Model file for the job. Use its own axes, mm. A direction names the side the tool comes from. Coordinates: 2 decimals unless noted, no trailing zeros. Loops run counter-clockwise (first coordinate to the right, second up) from the corner with the lowest first, then second, coordinate; pieces in that order, holes last. Notation, with made-up numbers: (-39.75, -15) -> (-34.75, -15) arc R14 cw to (-34.75, 12) -> close; hole circle Ø1 at (7.25, 77.5). An arc over 180 degrees is marked (long way). Use one line per item in the form item = value.
```python
from build123d import *

# Parameters (mm, degrees)
BOSS_EXTRUDE1_DEPTH             = 15.875
SKETCH2_R                       = 4.7625
CUT_EXTRUDE1_DEPTH              = 8
SKETCH3_R                       = 4.7625
CUT_EXTRUDE2_DEPTH              = 8
CUT_EXTRUDE3_DEPTH              = 60.905780189
BOSS_EXTRUDE2_REACH             = 62.821
BOSS_EXTRUDE2_DIRECTION_2_DEPTH = 31.75
SKETCH6_R                       = 4.7625
CUT_EXTRUDE4_DEPTH              = 83.269033521
CUT_EXTRUDE5_DEPTH              = 31.75
BOSS_EXTRUDE4_DEPTH             = 31.75
CUT_EXTRUDE6_DEPTH              = 93.319424063
BOSS_EXTRUDE5_DEPTH             = 12.7
BOSS_EXTRUDE6_DEPTH             = 6.35
CUT_EXTRUDE7_DEPTH              = 71.05833388
CUT_EXTRUDE8_REACH              = 78.805
SKETCH15_R                      = 2.25
CUT_EXTRUDE9_DEPTH              = 44.45
CUT_EXTRUDE10_DEPTH             = 12.7
SKETCH21_W                      = 12.513073453
SKETCH21_H                      = 19.05
CUT_EXTRUDE11_DEPTH             = 69.753972493


with BuildPart() as part:
    # Sketch1 → Boss-Extrude1 (new, symmetric)
    with BuildSketch(Plane(origin=(0, 0, 0), x_dir=(1, 0, 0), z_dir=(0, 1, 0))):
        Polygon((-35.921024484, 0), (0, 35.921024484), (35.921024484, 0), (0, -35.921024484), align=None)
    extrude(amount=BOSS_EXTRUDE1_DEPTH, both=True)

    # Sketch2 → Cut-Extrude1 (cut)
    with BuildSketch(Plane(origin=(17.960512242, 0, 17.960512242), x_dir=(0.7071067811865476, 0, -0.7071067811865476), z_dir=(0.7071067811865476, 0, 0.7071067811865476))):
        Circle(SKETCH2_R)
    extrude(amount=-CUT_EXTRUDE1_DEPTH, mode=Mode.SUBTRACT)

    # Sketch3 → Cut-Extrude2 (cut)
    with BuildSketch(Plane(origin=(-17.960512242, 0, 17.960512242), x_dir=(0.7071067811865472, 0, 0.7071067811865478), z_dir=(-0.7071067811865478, 0, 0.7071067811865472))):
        Circle(SKETCH3_R)
    extrude(amount=-CUT_EXTRUDE2_DEPTH, mode=Mode.SUBTRACT)

    # Sketch4 → Cut-Extrude3 (cut, through all)
    with BuildSketch(Plane(origin=(0, 15.875, 0), x_dir=(1, 0, 0), z_dir=(0, 1, 0))):
        Polygon((25.4, 10.521024484), (-25.4, 10.521024484), (0, 35.921024484), align=None)
    extrude(amount=-CUT_EXTRUDE3_DEPTH, mode=Mode.SUBTRACT)

    # Boss-Extrude2: up to this face of the body (flat: up to its plane)
    boss_extrude2_end = Plane(part.part.faces().sort_by_distance((30.660512242, 0, -5.260512242))[0])
    # Sketch5 → Boss-Extrude2 (add, up to the picked face)
    with BuildSketch(Plane(origin=(0, 0, -10.521024484), x_dir=(-1, 0, 0), z_dir=(0, 0, -1)), mode=Mode.PRIVATE) as boss_extrude2_sk1:
        Polygon((-35.921024484, 15.875), (-35.921024484, -15.875), (39.135030454, -15.875), (27.578975516, 15.875), align=None)
    boss_extrude2_tool1 = split(extrude(boss_extrude2_sk1.sketch, amount=-BOSS_EXTRUDE2_REACH, mode=Mode.PRIVATE), bisect_by=boss_extrude2_end, keep=Keep.BOTH, mode=Mode.PRIVATE)
    add(boss_extrude2_tool1.solids().sort_by(Axis((1.201693, -0.441343, -10.521024), (0, 0, 1)))[0])

    # Sketch5 → Boss-Extrude2 direction 2 (add)
    with BuildSketch(Plane(origin=(0, 0, -10.521024484), x_dir=(-1, 0, 0), z_dir=(0, 0, -1))):
        Polygon((-35.921024484, 15.875), (-35.921024484, -15.875), (39.135030454, -15.875), (27.578975516, 15.875), align=None)
    extrude(amount=BOSS_EXTRUDE2_DIRECTION_2_DEPTH)

    # Sketch6 → Cut-Extrude4 (cut, through all)
    with BuildSketch(Plane(origin=(-29.45497488, 10.720734107, 0), x_dir=(0, 0, 1), z_dir=(-0.9396926207859072, 0.3420201433256724, 0))):
        with Locations(Location((-26.396024484, -11.408766942, 0), (0, 0, 270))):
            Circle(SKETCH6_R)
    extrude(amount=-CUT_EXTRUDE4_DEPTH, mode=Mode.SUBTRACT)

    # Sketch7 → Cut-Extrude5 (cut)
    with BuildSketch(Plane(origin=(0, 0, -42.271024484), x_dir=(-1, 0, 0), z_dir=(0, 0, -1))):
        Polygon((20.821446661, 15.875), (32.377501598, -15.875), (-35.921024484, -15.875), (-35.921024484, 15.875), align=None)
    extrude(amount=-CUT_EXTRUDE5_DEPTH, mode=Mode.SUBTRACT)

    # Sketch9 → Boss-Extrude4 (add)
    with BuildSketch(Plane.XZ.offset(15.875)):
        Polygon((-25.4, -10.521024484), (-35.921024484, 0), (-46.442048969, -10.521024484), align=None)
    extrude(amount=-BOSS_EXTRUDE4_DEPTH)

    # Sketch10 → Cut-Extrude6 (cut, through all)
    with BuildSketch(Plane(origin=(0, 0, -42.271024484), x_dir=(-1, 0, 0), z_dir=(0, 0, -1))):
        Polygon((46.442048969, -15.875), (46.442048969, 15.875), (27.578975516, 15.875), (39.135030454, -15.875), align=None)
    extrude(amount=-CUT_EXTRUDE6_DEPTH, mode=Mode.SUBTRACT)

    # Sketch11 → Boss-Extrude5 (add)
    with BuildSketch(Plane.XZ.offset(15.875)):
        Polygon((-32.377501598, -10.521024484), (-39.135030454, -10.521024484), (-39.135030454, -3.214005969), (0, 35.921024484), (35.921024484, 0), (35.921024484, -10.521024484), align=None)
    extrude(amount=BOSS_EXTRUDE5_DEPTH)

    # Sketch12 → Boss-Extrude6 (add)
    with BuildSketch(Plane.XZ.offset(28.575)):
        Polygon((35.921024484, -10.521024484), (35.921024484, 0), (0, 35.921024484), (-39.135030454, -3.214005969), (-39.135030454, -42.271024484), (35.921024484, -42.271024484), align=None)
    extrude(amount=BOSS_EXTRUDE6_DEPTH)

    # Sketch14 → Cut-Extrude7 (cut, through all)
    with BuildSketch(Plane(origin=(0, 0, -10.521024484), x_dir=(-1, 0, 0), z_dir=(0, 0, -1))):
        Polygon((36.999923574, -28.575), (20.821446661, 15.875), (5.050498603, 15.875), (21.228975516, -28.575), (21.228975516, -34.925), (39.135030454, -34.925), (39.135030454, -28.575), align=None)
    extrude(amount=CUT_EXTRUDE7_DEPTH, mode=Mode.SUBTRACT)

    # Sketch15 → Cut-Extrude8 (cut, up to next)
    with BuildSketch(Plane.XZ.offset(34.925), mode=Mode.PRIVATE) as cut_extrude8_sk1:
        with Locations(Location((32.346024484, -36.396024484, 0), (0, 0, 270))):
            Circle(SKETCH15_R)
    cut_extrude8_tool1 = extrude(cut_extrude8_sk1.sketch, amount=-CUT_EXTRUDE8_REACH, mode=Mode.PRIVATE) & part.part
    # Sketch15 → Cut-Extrude8 (cut, up to next)
    with BuildSketch(Plane.XZ.offset(34.925), mode=Mode.PRIVATE) as cut_extrude8_sk2:
        with Locations(Location((32.346024484, -16.396024484, 0), (0, 0, 270))):
            Circle(SKETCH15_R)
    cut_extrude8_tool2 = extrude(cut_extrude8_sk2.sketch, amount=-CUT_EXTRUDE8_REACH, mode=Mode.PRIVATE) & part.part
    # Sketch15 → Cut-Extrude8 (cut, up to next)
    with BuildSketch(Plane.XZ.offset(34.925), mode=Mode.PRIVATE) as cut_extrude8_sk3:
        with Locations(Location((-17.653975516, -16.396024484, 0), (0, 0, 270))):
            Circle(SKETCH15_R)
    cut_extrude8_tool3 = extrude(cut_extrude8_sk3.sketch, amount=-CUT_EXTRUDE8_REACH, mode=Mode.PRIVATE) & part.part
    # Sketch15 → Cut-Extrude8 (cut, up to next)
    with BuildSketch(Plane.XZ.offset(34.925), mode=Mode.PRIVATE) as cut_extrude8_sk4:
        with Locations(Location((-17.653975516, -36.396024484, 0), (0, 0, 270))):
            Circle(SKETCH15_R)
    cut_extrude8_tool4 = extrude(cut_extrude8_sk4.sketch, amount=-CUT_EXTRUDE8_REACH, mode=Mode.PRIVATE) & part.part
    add(cut_extrude8_tool1.solids().sort_by_distance((32.346024, -34.925, -36.396024))[0], mode=Mode.SUBTRACT)
    add(cut_extrude8_tool2.solids().sort_by_distance((32.346024, -34.925, -16.396024))[0], mode=Mode.SUBTRACT)
    add(cut_extrude8_tool3.solids().sort_by_distance((-17.653976, -34.925, -16.396024))[0], mode=Mode.SUBTRACT)
    add(cut_extrude8_tool4.solids().sort_by_distance((-17.653976, -34.925, -36.396024))[0], mode=Mode.SUBTRACT)

    # Sketch17 → Cut-Extrude9 (cut)
    with BuildSketch(Plane(origin=(0, 15.875, 0), x_dir=(1, 0, 0), z_dir=(0, 1, 0))):
        Polygon((-20.821446661, 10.521024484), (-20.821446661, -6.119321703), (0, -26.940768363), (29.163495629, 2.222727266), (29.163495629, 10.521024484), align=None)
    extrude(amount=-CUT_EXTRUDE9_DEPTH, mode=Mode.SUBTRACT)

    # Sketch20 → Cut-Extrude10 (cut)
    with BuildSketch(Plane(origin=(0, 0, -10.521024484), x_dir=(-1, 0, 0), z_dir=(0, 0, -1))):
        Polygon((21.228975516, -28.575), (21.228975516, -34.925), (39.135030454, -34.925), (39.135030454, -15.875), (32.377501598, -15.875), (20.821446661, 15.875), (20.821446661, -28.575), align=None)
    extrude(amount=-CUT_EXTRUDE10_DEPTH, mode=Mode.SUBTRACT)

    # Sketch21 → Cut-Extrude11 (cut, through all)
    with BuildSketch(Plane(origin=(0, 0, 2.178975516), x_dir=(-1, 0, 0), z_dir=(0, 0, -1))):
        with Locations((27.485512243, -25.4)):
            Rectangle(SKETCH21_W, SKETCH21_H)
    extrude(amount=-CUT_EXTRUDE11_DEPTH, mode=Mode.SUBTRACT)


solid = part.part
```
Q1. Band-saw the part on C-C, the plane y = -17.5. Write the cut outline in (x, z), and give its area (3 significant figures).
Result:
outline = (-21.23, 2.18) -> (-20.82, 2.18) -> (-20.82, 6.12) -> (0, 26.94) -> (29.16, -2.22) -> (29.16, -10.52) -> (35.92, -10.52) -> (35.92, 0) -> (0, 35.92) -> (-21.23, 14.69) -> close
area = 548 mm2
Q2. Mould opens along X. For faces 4 (the face through (15.02, -4.65, 16.48)), 5 (the face through (18.21, -9.17, 17.71)), 6 (the face through (-30, 0, -42.271)), 7 (the face through (-21.229, -29, -7)) say: released by +X, released by -X, zero draft, split by the parting line, or undercut.
Result:
face_4 = undercut
face_5 = released by +X
face_6 = zero draft
face_7 = released by -X
Q3. Band-saw the part on B-B, the plane y = -32. Write the cut outline in (x, z), and give its area (3 significant figures).
Result:
outline = (-21.23, -42.27) -> (35.92, -42.27) -> (35.92, 0) -> (0, 35.92) -> (-21.23, 14.69) -> close; hole circle Ø4.5 at (-17.65, -36.4); hole circle Ø4.5 at (-17.65, -16.4); hole circle Ø4.5 at (32.35, -36.4); hole circle Ø4.5 at (32.35, -16.4)
area = 3,530 mm2
Q4. Pin check, flat tips, straight feed: pin 1 Ø1.5 at (x, y) = (-29, 10) entering from +Z; pin 2 Ø6 at (x, z) = (23, -3.5) entering from +Y (3 decimals); pin 3 Ø6.5 at (y, z) = (-2, -7.5) entering from -X; pin 4 Ø3.5 at (x, z) = (32.35, -16.4) entering from +Y. Stop position of each tip, or through.
Result:
pin_1 = 7.67
pin_2 = -28.575
pin_3 = -35.27
pin_4 = through
Q5. Band-saw the part on D-D, the plane x = -6. Write the cut outline in (y, z) (3 decimals), and give its area (3 significant figures).
Result:
outline = (-34.925, -42.271) -> (-28.575, -42.271) -> (-28.575, 20.941) -> (15.875, 20.941) -> (15.875, 29.921) -> (-34.925, 29.921) -> close
area = 858 mm2
Q6. Wall check: line 1 along Y through (x, z) = (-13, 11) (3 decimals); line 2 along X through (y, z) = (-32, -10.5); line 3 along X through (y, z) = (-3, 18.5). Give the ranges that are in metal, low to high.
Result:
line_1 = -34.925 to -28.575
line_2 = -21.23 to 35.92
line_3 = -13.27 to -8.44, 8.44 to 13.27
Q7. Which spindle directions (+Z, -Z, +X, -X, +Y, -Y) get a long thin tool onto all of the face, cutting with end or side? Do faces 1 (the face through (14.38, -6.04, 12.56)), 2 (the face through (-33, -15.875, -14)), 3 (the face through (32, -6, -10.521)). Say none if no direction does.
Result:
face_1 = -Z, +Y
face_2 = +Z, -Z, -X, -Y
face_3 = -Z, +X, +Y
Q8. Band-saw the part on A-A, the plane z = -7. Write the cut outline in (x, y) (1 decimal), and give its area (3 significant figures).
Result:
outline = (-39.1, -15.9) -> (-32.4, -15.9) -> (-20.8, 15.9) -> (-27.6, 15.9) -> close; (-21.2, -34.9) -> (35.9, -34.9) -> (35.9, 15.9) -> (29.2, 15.9) -> (29.2, -28.6) -> (-21.2, -28.6) -> close
area = 878 mm2
